Read the model definition and answer for the solid it produces. Units are mm, in the model's axes. Face numbers are marked on the shaded views. A direction names the side the tool comes from. Give positions to 0.01 mm unless a question says otherwise; leave off trailing zeros. Order: outer loops, then holes, each group sorted by start corner. A loop starts at its lowest first (then second) coordinate and runs counter-clockwise, first axis right, second up. Notation, with made-up numbers: M 24,-28 L 66,-28 A25 cw 66,-6 Z; hole C 88,65 d5. An arc over 180 degrees is marked long. One line per item, written item: value.
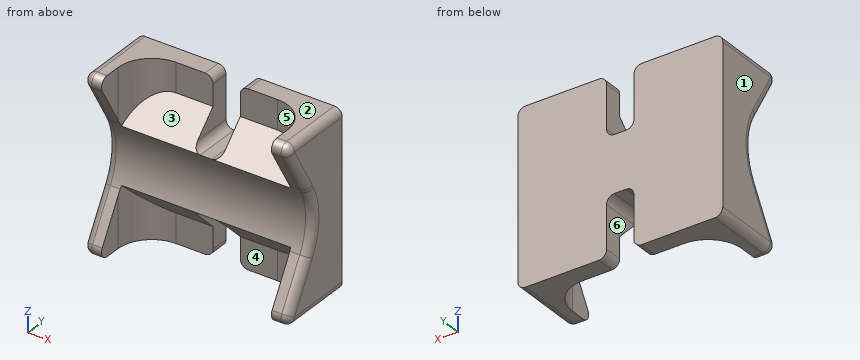
from build123d import *

# Parameters (mm, degrees)
SKETCH23_W          = 26.67
SKETCH23_H          = 22.606
BOSS_EXTRUDE8_DEPTH = 13.208
CUT_EXTRUDE1_DEPTH  = 7.62
SKETCH27_R          = 8.128
CUT_EXTRUDE3_DEPTH  = 38.1
CUT_EXTRUDE4_DEPTH  = 76.2
CHAMFER1_SIZE       = 3.81
FILLET1_R           = 1.016
FILLET2_R           = 1.016
FILLET4_R           = 1.016


with BuildPart() as part:
    # Sketch23 → Boss-Extrude8 (new body)
    with BuildSketch(Plane(origin=(0, 13.462, 0), x_dir=(1, 0, 0), z_dir=(0, 1, 0))):
        with Locations((0, 12.7)):
            Rectangle(SKETCH23_W, SKETCH23_H)
    extrude(amount=-BOSS_EXTRUDE8_DEPTH)

    # Sketch25 → Cut-Extrude1 (cut)
    with BuildSketch(Plane(origin=(0, 0, -24.003), x_dir=(-1, 0, 0), z_dir=(0, 0, -1))):
        with BuildLine():
            Line((1.778, 13.462), (1.778, 11.045488249))
            Line((1.778, 11.045488249), (6.600488249, 11.045488249))
            ThreePointArc((6.600488249, 11.045488249), (9.743577891, 9.743577891), (11.045488249, 6.600488249))
            Line((11.045488249, 6.600488249), (11.045488249, 0.254))
            Line((11.045488249, 0.254), (-11.045488249, 0.254))
            Line((-11.045488249, 0.254), (-11.045488249, 6.600488249))
            ThreePointArc((-11.045488249, 6.600488249), (-9.743577891, 9.743577891), (-6.600488249, 11.045488249))
            Line((-6.600488249, 11.045488249), (-1.778, 11.045488249))
            Line((-1.778, 11.045488249), (-1.778, 13.462))
            ThreePointArc((-1.778, 13.462), (0, 15.24), (1.778, 13.462))
        make_face()
    cut_extrude1 = extrude(amount=-CUT_EXTRUDE1_DEPTH, mode=Mode.SUBTRACT)

    # Sketch27 → Cut-Extrude3 (cut, symmetric)
    with BuildSketch(Plane(origin=(0, 0, 0), x_dir=(0, 0, -1), z_dir=(1, 0, 0))):
        with Locations((12.7, 0)):
            Circle(SKETCH27_R)
    extrude(amount=CUT_EXTRUDE3_DEPTH, both=True, mode=Mode.SUBTRACT)

    # Sketch28 → Cut-Extrude4 (cut)
    with BuildSketch(Plane(origin=(13.335, 0, 0), x_dir=(0, 0, -1), z_dir=(1, 0, 0))):
        with BuildLine():
            Line((1.397, 2.859615883), (8.636, 7.039054482))
            ThreePointArc((8.636, 7.039054482), (12.7, 8.128), (16.764, 7.039054482))
            Line((16.764, 7.039054482), (24.003, 2.859615883))
            Line((24.003, 2.859615883), (24.003, 0.254))
            Line((24.003, 0.254), (1.397, 0.254))
            Line((1.397, 0.254), (1.397, 2.859615883))
        make_face()
    extrude(amount=-CUT_EXTRUDE4_DEPTH, mode=Mode.SUBTRACT)

    # Mirror1: Cut-Extrude1 across plane
    add(cut_extrude1.mirror(Plane.XY.offset(-12.7)), mode=Mode.SUBTRACT)

    # Chamfer1
    # the kernel refuses this chamfer: 3.81 mm, written as the material it adds along each edge
    with BuildSketch(Plane(origin=(8.020112184, 11.045488249, -16.383), x_dir=(0, -1, 0), z_dir=(-1, 0, 0))) as chamfer1_piece_1_section:
        Polygon((CHAMFER1_SIZE, 0), (0, -CHAMFER1_SIZE), (0, 0), align=None)
    chamfer1_piece_1 = extrude(amount=24.418712617, mode=Mode.PRIVATE)
    chamfer1_piece_1 = split(chamfer1_piece_1, bisect_by=Plane(origin=(1.778, 11.045488249, -16.383), z_dir=(1, 0, 0)), keep=Keep.TOP, mode=Mode.PRIVATE)
    chamfer1_piece_1 = chamfer1_piece_1 - Plane(origin=(8.020112184, 0, -12.7), x_dir=(0, 0, -1), z_dir=(1, 0, 0)) * Cylinder(8.128, 65, mode=Mode.PRIVATE)
    add(chamfer1_piece_1)
    with BuildSketch(Plane(origin=(-1.778, 11.045488249, -16.383), x_dir=(0, -1, 0), z_dir=(-1, 0, 0))) as chamfer1_piece_2_section:
        Polygon((CHAMFER1_SIZE, 0), (0, -CHAMFER1_SIZE), (0, 0), align=None)
    chamfer1_piece_2 = extrude(amount=14.620600433, mode=Mode.PRIVATE)
    chamfer1_piece_2 = split(chamfer1_piece_2, bisect_by=Plane(origin=(-13.335, 11.045488249, -16.383), z_dir=(1, 0, 0)), keep=Keep.TOP, mode=Mode.PRIVATE)
    chamfer1_piece_2 = chamfer1_piece_2 - Plane(origin=(-1.778, 0, -12.7), x_dir=(0, 0, -1), z_dir=(1, 0, 0)) * Cylinder(8.128, 45, mode=Mode.PRIVATE)
    add(chamfer1_piece_2)
    with BuildSketch(Plane(origin=(16.398600433, 11.045488249, -16.383), x_dir=(0, -1, 0), z_dir=(-1, 0, 0))) as chamfer1_piece_3_section:
        Polygon((CHAMFER1_SIZE, 0), (0, -CHAMFER1_SIZE), (0, 0), align=None)
    chamfer1_piece_3 = extrude(amount=14.620600433, mode=Mode.PRIVATE)
    chamfer1_piece_3 = split(chamfer1_piece_3, bisect_by=Plane(origin=(13.335, 11.045488249, -16.383), z_dir=(-1, 0, 0)), keep=Keep.TOP, mode=Mode.PRIVATE)
    chamfer1_piece_3 = chamfer1_piece_3 - Plane(origin=(16.398600433, 0, -12.7), x_dir=(0, 0, -1), z_dir=(1, 0, 0)) * Cylinder(8.128, 45, mode=Mode.PRIVATE)
    add(chamfer1_piece_3)
    with BuildSketch(Plane(origin=(16.398600433, 11.045488249, -16.383), x_dir=(0, -1, 0), z_dir=(-1, 0, 0))) as chamfer1_piece_4_section:
        Polygon((CHAMFER1_SIZE, 0), (0, -CHAMFER1_SIZE), (0, 0), align=None)
    chamfer1_piece_4 = extrude(amount=24.418712617, mode=Mode.PRIVATE)
    chamfer1_piece_4 = split(chamfer1_piece_4, bisect_by=Plane(origin=(-1.778, 11.045488249, -16.383), z_dir=(-1, 0, 0)), keep=Keep.TOP, mode=Mode.PRIVATE)
    chamfer1_piece_4 = chamfer1_piece_4 - Plane(origin=(16.398600433, 0, -12.7), x_dir=(0, 0, -1), z_dir=(1, 0, 0)) * Cylinder(8.128, 65, mode=Mode.PRIVATE)
    add(chamfer1_piece_4)
    with BuildSketch(Plane(origin=(8.020112184, 11.045488249, -9.017), x_dir=(0, 0, 1), z_dir=(-1, 0, 0))) as chamfer1_piece_5_section:
        Polygon((CHAMFER1_SIZE, 0), (0, -CHAMFER1_SIZE), (0, 0), align=None)
    chamfer1_piece_5 = extrude(amount=24.418712617, mode=Mode.PRIVATE)
    chamfer1_piece_5 = split(chamfer1_piece_5, bisect_by=Plane(origin=(1.778, 11.045488249, -9.017), z_dir=(1, 0, 0)), keep=Keep.TOP, mode=Mode.PRIVATE)
    chamfer1_piece_5 = chamfer1_piece_5 - Plane(origin=(8.020112184, 0, -12.7), x_dir=(0, 0, -1), z_dir=(1, 0, 0)) * Cylinder(8.128, 65, mode=Mode.PRIVATE)
    add(chamfer1_piece_5)
    with BuildSketch(Plane(origin=(-1.778, 11.045488249, -9.017), x_dir=(0, 0, 1), z_dir=(-1, 0, 0))) as chamfer1_piece_6_section:
        Polygon((CHAMFER1_SIZE, 0), (0, -CHAMFER1_SIZE), (0, 0), align=None)
    chamfer1_piece_6 = extrude(amount=14.620600433, mode=Mode.PRIVATE)
    chamfer1_piece_6 = split(chamfer1_piece_6, bisect_by=Plane(origin=(-13.335, 11.045488249, -9.017), z_dir=(1, 0, 0)), keep=Keep.TOP, mode=Mode.PRIVATE)
    chamfer1_piece_6 = chamfer1_piece_6 - Plane(origin=(-1.778, 0, -12.7), x_dir=(0, 0, -1), z_dir=(1, 0, 0)) * Cylinder(8.128, 45, mode=Mode.PRIVATE)
    add(chamfer1_piece_6)
    with BuildSketch(Plane(origin=(16.398600433, 11.045488249, -9.017), x_dir=(0, -1, 0), z_dir=(-1, 0, 0))) as chamfer1_piece_7_section:
        Polygon((CHAMFER1_SIZE, 0), (0, CHAMFER1_SIZE), (0, 0), align=None)
    chamfer1_piece_7 = extrude(amount=14.620600433, mode=Mode.PRIVATE)
    chamfer1_piece_7 = split(chamfer1_piece_7, bisect_by=Plane(origin=(13.335, 11.045488249, -9.017), z_dir=(-1, 0, 0)), keep=Keep.TOP, mode=Mode.PRIVATE)
    chamfer1_piece_7 = chamfer1_piece_7 - Plane(origin=(16.398600433, 0, -12.7), x_dir=(0, 0, -1), z_dir=(1, 0, 0)) * Cylinder(8.128, 45, mode=Mode.PRIVATE)
    add(chamfer1_piece_7)
    with BuildSketch(Plane(origin=(16.398600433, 11.045488249, -9.017), x_dir=(0, -1, 0), z_dir=(-1, 0, 0))) as chamfer1_piece_8_section:
        Polygon((CHAMFER1_SIZE, 0), (0, CHAMFER1_SIZE), (0, 0), align=None)
    chamfer1_piece_8 = extrude(amount=24.418712617, mode=Mode.PRIVATE)
    chamfer1_piece_8 = split(chamfer1_piece_8, bisect_by=Plane(origin=(-1.778, 11.045488249, -9.017), z_dir=(-1, 0, 0)), keep=Keep.TOP, mode=Mode.PRIVATE)
    chamfer1_piece_8 = chamfer1_piece_8 - Plane(origin=(16.398600433, 0, -12.7), x_dir=(0, 0, -1), z_dir=(1, 0, 0)) * Cylinder(8.128, 65, mode=Mode.PRIVATE)
    add(chamfer1_piece_8)

    # Fillet1
    fillet1_edges = [part.edges().sort_by_distance(p)[0] for p in [
        (12.190244124, 2.859615883, -1.397),
        (-12.190244124, 2.859615883, -24.003),
        (12.190244124, 2.859615883, -24.003),
        (-12.190244124, 2.859615883, -1.397),
    ]]
    fillet(fillet1_edges, radius=FILLET1_R)

    # Fillet2
    fillet2_edges = [part.edges().sort_by_distance(p)[0] for p in [
        (1.778, 10.353840564, -9.017),
        (-1.778, 10.353840564, -9.017),
        (1.778, 12.253744124, -1.397),
        (-1.778, 12.253744124, -1.397),
        (1.778, 10.353840564, -16.383),
        (-1.778, 10.353840564, -16.383),
        (-1.778, 12.253744124, -24.003),
        (1.778, 12.253744124, -24.003),
    ]]
    fillet(fillet2_edges, radius=FILLET2_R)

    # Fillet4
    fillet4_edges = [part.edges().sort_by_distance(p)[0] for p in [
        (13.335, 9.040689752, -1.397),
        (13.335, 5.389276088, -5.7785),
        (13.335, 5.389276088, -19.6215),
        (13.335, 9.040689752, -24.003),
        (13.335, 3.739497694, -23.495),
        (13.335, 3.739497694, -1.905),
        (-13.335, 9.040689752, -1.397),
        (-13.335, 9.040689752, -24.003),
        (-13.335, 3.739497694, -23.495),
        (-13.335, 3.739497694, -1.905),
        (13.335, 8.128, -12.7),
        (-13.335, 8.128, -12.7),
        (-13.335, 5.389276088, -19.6215),
        (-13.335, 5.389276088, -5.7785),
    ]]
    fillet(fillet4_edges, radius=FILLET4_R)


solid = part.part
1) Find section C-C, the plane y = 10. Write down the section's boundary in (x, z) (3 decimals), plus the area to 3 significant figures.
Reported:
outline: M -13.335,-22.987 A1.016 ccw -12.319,-24.003 L -9.464,-24.003 L -9.464,-19.148 L -1.778,-19.148 L -1.778,-17.399 A1.016 cw -0.762,-16.383 L 0.762,-16.383 A1.016 cw 1.778,-17.399 L 1.778,-19.148 L 9.464,-19.148 L 9.464,-24.003 L 12.319,-24.003 A1.016 ccw 13.335,-22.987 L 13.335,-2.413 A1.016 ccw 12.319,-1.397 L 9.464,-1.397 L 9.464,-6.252 L 1.778,-6.252 L 1.778,-8.001 A1.016 cw 0.762,-9.017 L -0.762,-9.017 A1.016 cw -1.778,-8.001 L -1.778,-6.252 L -9.464,-6.252 L -9.464,-1.397 L -12.319,-1.397 A1.016 ccw -13.335,-2.413 Z
area: 399 mm^2
2) Which of the six approach directions +Z, -Z, +X, -X, +Y, -Y give full straight-line access (tool end or side, diameter ignored) to the marked faces 4, 5 and 6?
Reported:
face 4: -Z, -Y
face 5: +Z, -Y
face 6: -Z, +Y, -Y
3) Find section A-A, the plane x = 6.25. Write down the section's boundary in (y, z), plus the area to 3 significant figures.
Reported:
outline: M 7.24,-16.39 L 11.05,-20.19 L 11.05,-24 L 13.46,-24 L 13.46,-1.4 L 11.05,-1.4 L 11.05,-5.21 L 7.24,-9.01 A8.13 cw Z
area: 92.8 mm^2
4) Consider probe 1 along X at (y, z) = (6.75, -21) (3 decimals); probe 2 along Z at (x, y) = (4, 8.25); probe 3 along Y at (x, z) = (-2.75, -22.5). Determine where each line is inside the solid, lowest interval first.
Reported:
probe 1: x = -13.335 to -11.043, 11.043 to 13.335
probe 2: z = -17.4 to -8
probe 3: y = 11.05 to 13.46
5) Find section D-D, the plane x = -8.75. Write down the section's boundary in (y, z), plus the area to 3 significant figures.
Reported:
outline: M 7.24,-16.39 L 10.49,-19.64 L 10.49,-24 L 13.46,-24 L 13.46,-1.4 L 10.49,-1.4 L 10.49,-5.76 L 7.24,-9.01 A8.13 cw Z
area: 97.3 mm^2
6) Each of these flat-tipped pins is pushed along its axis until it touches: pin 1 Ø1.1 at (x, z) = (3.5, -21.5) entering from -Y; pin 2 Ø0.5 at (x, y) = (0, 12) entering from +Z; pin 3 Ø3 at (x, z) = (-3.5, -4) entering from -Y. Where does it stop, or does it pass through?
Reported:
pin 1: stops at y = 11.05
pin 2: stops at z = -9.02
pin 3: stops at y = 10.75
7) Find section B-B, the plane y = 11.5. Write down the section's boundary in (x, z) (3 decimals), plus the area to 3 significant figures.
Reported:
outline: M -13.335,-22.987 A1.016 ccw -12.319,-24.003 L -2.794,-24.003 A1.016 ccw -1.778,-22.987 L -1.778,-17.399 A1.016 cw -0.762,-16.383 L 0.762,-16.383 A1.016 cw 1.778,-17.399 L 1.778,-22.987 A1.016 ccw 2.794,-24.003 L 12.319,-24.003 A1.016 ccw 13.335,-22.987 L 13.335,-2.413 A1.016 ccw 12.319,-1.397 L 2.794,-1.397 A1.016 ccw 1.778,-2.413 L 1.778,-8.001 A1.016 cw 0.762,-9.017 L -0.762,-9.017 A1.016 cw -1.778,-8.001 L -1.778,-2.413 A1.016 ccw -2.794,-1.397 L -12.319,-1.397 A1.016 ccw -13.335,-2.413 Z
area: 548 mm^2
8) Determine the mould class of the marked faces 1, 2 and 3 for opening direction X: +X half, -X half, draft (parallel to the pull), parting line (faces both ways), or undercut.
Reported:
face 1: -X half
face 2: draft
face 3: undercut
